Autodesk Inventor part; units mm, degrees
ref_plane "Work Plane1" through (-55, 40, 80) normal (0, 0, 1) x (1, 0, 0)
ref_plane "YZ Plane" through (0, 0, 0) normal (1, 0, 0) x (0, 1, 0)
ref_plane "XZ Plane" through (0, 0, 0) normal (0, 1, 0) x (-1, 0, 0)
sketch "Sketch1" plane through (0, 0, 0) normal (0, 1, 0) x (-1, 0, 0)
  line L0 (75, -100) -> (-75, -100)
  line L1 (-75, -100) -> (-75, 100)
  line L2 (-75, 100) -> (75, 100)
  line L3 (75, 100) -> (75, -100)
  line L4 (75, -100) -> (-75, 100) construction
  line L5 (-75, -100) -> (75, 100) construction
  line L6 (55, 80) -> (-55, 80)
  line L7 (-60, 75) -> (-60, 25)
  line L8 (-55, 20) -> (55, 20)
  line L9 (60, 25) -> (60, 75)
  line L10 (60, 80) -> (-60, 20) construction
  line L11 (-60, 80) -> (60, 20) construction
  circle A0 centre (38, -50.6667) radius 30
  circle A1 centre (38, -70.6667) radius 7.5
  circle A2 centre (55.3205, -60.6667) radius 7.5
  circle A3 centre (55.3205, -40.6667) radius 7.5
  circle A4 centre (38, -30.6667) radius 7.5
  circle A5 centre (20.6795, -40.6667) radius 7.5
  circle A6 centre (20.6795, -60.6667) radius 7.5
  arc A7 (55, 20) -> (60, 25) centre (55, 25) ccw
  arc A8 (60, 75) -> (55, 80) centre (55, 75) ccw
  arc A9 (-55, 80) -> (-60, 75) centre (-55, 75) ccw
  arc A10 (-60, 25) -> (-55, 20) centre (-55, 25) ccw
  arc A11 (-42, -64.1421) -> (-41.9301, -64.1667) centre (-37, -50) ccw
  arc A12 (-22, -45) -> (-22, -55) centre (-22, -50) ccw
  arc A13 (-7, -55) -> (-7, -45) centre (-7, -50) ccw
  line L12 (-7, -45) -> (-22, -45)
  line L13 (-7, -55) -> (-22, -55)
  line L14 (-42, -20) -> (-42, -35)
  arc A14 (-42, -35) -> (-32, -35) centre (-37, -35) ccw
  line L15 (-32, -20) -> (-32, -35)
  arc A15 (-32, -20) -> (-42, -20) centre (-37, -20) ccw
  line L16 (-67, -55) -> (-52, -55)
  arc A16 (-52, -55) -> (-52, -45) centre (-52, -50) ccw
  line L17 (-67, -45) -> (-52, -45)
  arc A17 (-67, -45) -> (-67, -55) centre (-67, -50) ccw
  line L18 (-32, -80) -> (-32, -65)
  arc A18 (-32, -65) -> (-42, -65) centre (-37, -65) ccw
  line L19 (-42, -80) -> (-42, -65)
  arc A19 (-42, -80) -> (-32, -80) centre (-37, -80) ccw
  point P0 (0, 0)
  point P1 (0, 50)
  dimension "d0" = 150
  dimension "d1" = 200
  dimension "d2" = 50
  dimension "d3" = 75
  dimension "d4" = 60
  dimension "d5" = 120
  dimension "d29" = 15
  dimension "d30" = 20
  dimension "d33" = 360
  dimension "d35" = 5
  dimension "d36" = 5
  dimension "d37" = 30
  dimension "d38" = 100
  dimension "d39" = 38
  dimension "d42" = 15
  dimension "d45" = 360
  dimension "d47" = 75
  dimension "d62" = 60
  dimension "d63" = 5
  dimension "d64" = 5
extrude "Extrusion1" add sketch "Sketch1" along normal blind 40 contours L0 L1 L2 L3
extrude "Extrusion2" add sketch "Sketch1" along normal blind 60 contours A8 L9 A7 L8 A10 L7 A9 L6
extrude "Extrusion3" add sketch "Sketch1" along normal blind 30 contours A0
extrude "Extrusion4" add sketch "Sketch1" along normal blind 35 contours L12 A13 L13 A12 | A15 L15 A14 L14 | A17 L17 A16 L16 | A19 L19 A18 L18
extrude "Extrusion5" add sketch "Sketch1" along normal blind 25 contours A1 | A2 | A3 | A4 | A5 | A6
ref_plane "Work Plane1" through (-55, 40, 80) normal (0, 0, 1) x (1, 0, 0)
sketch "Sketch2" plane through (-55, 40, 80) normal (0, 0, 1) x (1, 0, 0)
  line L0 (-5, 0) -> (-5, 20)
  line L1 (-5, 20) -> (121.275, 0)
  line L2 (-5, 20) -> (122.8491, 20) construction
  line L3 (121.275, 0) -> (121.275, 40.187)
  line L4 (122, 0) -> (127, 0)
  line L5 (121.275, 40.187) -> (-5, 40.187)
  line L6 (-5, 40.187) -> (-5, 20)
  point P0 (55, -40)
  dimension "d59" = 9
extrude "Extrusion6" cut sketch "Sketch2" against normal through all
properties part number "Tarefa 4" material "Glass"
The model under review builds one solid part; all positions refer to its coordinate system, in mm. Round coordinates to 2 decimals unless told otherwise and drop trailing zeros. Write each loop counter-clockwise with the first axis right and the second up, starting at its lowest first coordinate (ties: lowest second). Pieces come first, ordered by that corner, then holes. Notation, with made-up numbers: (89, 89.5) -> (135, 89.5) arc R14 cw to (135, 97.5) -> close; hole circle Ø11 at (45.25, -25.75). An arc over 180 degrees is marked (long way). Use CSV: the item, a comma, the result in double quotes.
Q1. To check wall thickness, follow probe 1 along Z at (x, y) = (-38, 29); probe 2 along Y at (x, z) = (66, 59.5); probe 3 along Z at (x, y) = (52, 39). State the ranges of each line that lie inside material, in increasing order. Write a range as [from, to].
Checks:
probe 1,"[-100, -78.17], [-63.17, -38.17], [-23.17, 100]"
probe 2,"[0, 40]"
probe 3,"[-100, -55], [-45, 100]"
Q2. Consider section C-C (y = 47). Give the boundary of the cut face in (x, z).
Checks:
outline,"(-60, 25) arc R5 ccw to (-55, 20) -> (22.08, 20) -> (22.08, 80) -> (-55, 80) arc R5 ccw to (-60, 75) -> close"
Q3. For pin 1 Ø0.5 at (y, z) = (40.5, 46.5) entering from +X; pin 2 Ø24 at (x, z) = (-38, -30.67) entering from +Y; pin 3 Ø4.5 at (x, z) = (-41.5, -30) entering from +Y, all flat-tipped, find the tip position at first contact; note any pin that passes through.
Checks:
pin 1,"x = 60"
pin 2,"y = 40"
pin 3,"y = 25"
Q4. Consider section A-A (z = 27.5). Give the boundary of the cut face in (x, y), then the cut area to 3 significant figures.
Checks:
outline,"(-75, 0) -> (75, 0) -> (75, 40) -> (60, 40) -> (60, 40.99) -> (-60, 60) -> (-60, 40) -> (-75, 40) -> close"
area,"7,260 mm²"
Q5. Mouldability with a two-part tool opening along Z and no side actions: class faces 1 (the flat face through (60, 37, -55)), 2 (the flat face through (-0.84, 50.63, 50.42)) as released by +Z, released by -Z, zero draft, split by the parting line, or undercut.
Checks:
face 1,"undercut"
face 2,"zero draft"
Q6. Consider section D-D (x = -57.5). Give the boundary of the cut face in (y, z).
Checks:
outline,"(0, -100) -> (40, -100) -> (40, -73.46) -> (30, -73.46) -> (30, -67.84) -> (25, -67.84) -> (25, -53.49) -> (30, -53.49) -> (30, -47.84) -> (25, -47.84) -> (25, -33.49) -> (30, -33.49) -> (30, -27.87) -> (40, -27.87) -> (40, 20.67) -> (59.6, 20.67) -> (59.6, 79.33) -> (40, 79.33) -> (40, 100) -> (0, 100) -> close"
Q7. Consider section B-B (x = 38). Give the boundary of the cut face in (y, z), then the cut area to 3 significant figures.
Checks:
outline,"(0, -100) -> (40, -100) -> (40, -84.9) -> (35, -84.9) -> (35, -60.1) -> (40, -60.1) -> (40, -39.9) -> (35, -39.9) -> (35, -15.1) -> (40, -15.1) -> (40, 20) -> (44.48, 20) -> (44.48, 80) -> (40, 80) -> (40, 100) -> (0, 100) -> close"
area,"8,020 mm²"
